from build123d import *

# Parameters (mm, degrees)
SKETCH1_R           = 13
BOSS_EXTRUDE1_DEPTH = 10
SKETCH3_R           = 17
BOSS_EXTRUDE2_DEPTH = 1
CUT_EXTRUDE2_DEPTH  = 27.438608133


with BuildPart() as part:
    # Sketch1 → Boss-Extrude1 (new body)
    with BuildSketch(Plane(origin=(0, 0, 0), x_dir=(1, 0, 0), z_dir=(0, 1, 0))):
        with Locations(Location((0, 0, 0), (0, 0, 270))):
            Circle(SKETCH1_R)
    extrude(amount=BOSS_EXTRUDE1_DEPTH)

    # Sketch2 → Cut-Revolve1 (revolve, cut)
    with BuildSketch(Plane(origin=(0, 0, 0), x_dir=(0, 0, -1), z_dir=(1, 0, 0)), mode=Mode.PRIVATE) as cut_revolve1_sk:
        Polygon((-13, 0), (-10.757403894, 10), (-13, 10), align=None)
    revolve(cut_revolve1_sk.sketch.rotate(Axis((0, 0, 0), (0, 1, 0)), 180), axis=Axis((0, 0, 0), (0, 1, 0)), mode=Mode.SUBTRACT)

    # Sketch3 → Boss-Extrude2 (add)
    with BuildSketch(Plane(origin=(0, 0, 0), x_dir=(-1, 0, 0), z_dir=(0, -1, 0))):
        with Locations(Location((0, 0, 0), (0, 0, 90))):
            Circle(SKETCH3_R)
    extrude(amount=BOSS_EXTRUDE2_DEPTH)

    # Sketch5 → Cut-Extrude2 (cut, through all)
    with BuildSketch(Plane(origin=(0, 10, 0), x_dir=(1, 0, 0), z_dir=(0, 1, 0))):
        with BuildLine():
            Line((1.322875656, 1.5), (-1.322875656, 1.5))
            ThreePointArc((-1.322875656, 1.5), (-0.822875656, -1.822875656), (2, 0))
            ThreePointArc((2, 0), (1.822875656, 0.822875656), (1.322875656, 1.5))
        make_face()
    extrude(amount=-CUT_EXTRUDE2_DEPTH, mode=Mode.SUBTRACT)


solid = part.part
Can you work these out from the model? Positions are in its coordinate system, mm. A direction names the side the tool comes from. Round coordinates to 2 decimals unless told otherwise and drop trailing zeros. Order: outer loops, then holes, each group sorted by start corner. A loop starts at its lowest first (then second) coordinate and runs counter-clockwise, first axis right, second up. Notation, with made-up numbers: M 26.25,12.25 L 34.25,12.25 A33 cw 34.25,48.25 Z; hole C 47,-20.5 d3. An arc over 180 degrees is marked long. Use a Markdown table: item, result.
1) I'm going to push flat-ended pins straight in: P1, Ø3.5, axis at x = 0, z = 0, coming from the +Y side; P2, Ø6, axis at y = 8.5, z = -9.5, coming from the +X side; P3, Ø3, axis at x = -0.5, y = 5.5, coming from the +Z side; P4, Ø1, axis at x = 9, y = 7, coming from the +Z side. Where does each tip first touch, or does it pass through?
Geometry says:
| item | result |
|---|---|
| P1 | stops at y = 10 |
| P2 | stops at x = 9.14 |
| P3 | stops at z = 12.1 |
| P4 | stops at z = 7.67 |
2) If I drill on line 1 along Y through (x, z) = (11, 9.5); line 2 along X through (y, z) = (5.5, 0.5); line 3 along Z through (x, y) = (9, 5), over which ranges is the centre line in solid material (lowest first)?
Geometry says:
| item | result |
|---|---|
| line 1 | y = -1 to 0 |
| line 2 | x = -11.76 to -1.94, 1.94 to 11.76 |
| line 3 | z = -7.75 to 7.75 |
3) Imagine slicing it at C-C (x = 13.5). List the corners of the cut face in (y, z) for me.
Geometry says:
| item | result |
|---|---|
| outline | M -1,-10.33 L 0,-10.33 L 0,10.33 L -1,10.33 Z |
4) On a 3-axis mill with a long thin cutter (end or side, diameter ignored), from which of +Z, -Z, +X, -X, +Y, -Y can I reach the whole of each face in a straight line? I mean faces 1 (the face through (-13, 0, 4)), 2 (the face through (-2.2, 10, -0.2)). Say none if no direction works.
Geometry says:
| item | result |
|---|---|
| face 1 | +Y |
| face 2 | +Z, -Z, +X, -X, +Y |
5) Imagine slicing it at A-A (x = 0). List the corners of the cut face in (y, z) for me, then the cut area to 3 significant figures.
Geometry says:
| item | result |
|---|---|
| outline | M -1,-17 L 0,-17 L 0,-13 L 10,-10.76 L 10,-1.5 L -1,-1.5 Z; M -1,2 L 10,2 L 10,10.76 L 0,13 L 0,17 L -1,17 Z |
| area | 233 mm² |
6) If we mould it in two halves opening along X, with no side actions, what happens to faces 3 (the face through (0, 5, -1.5)), 4 (the face through (-4, -1, 0)), 5 (the face through (16.855, -0.493, 2.213))? For each: +X half, -X half, draft (parallel to the pull), parting line (faces both ways), or undercut.
Geometry says:
| item | result |
|---|---|
| face 3 | undercut |
| face 4 | draft |
| face 5 | parting line |
7) Imagine slicing it at D-D (z = 14.5). List the corners of the cut face in (x, y) for me.
Geometry says:
| item | result |
|---|---|
| outline | M -8.87,-1 L 8.87,-1 L 8.87,0 L -8.87,0 Z |
8) Imagine slicing it at B-B (y = 5.5). List the corners of the cut face in (x, z) for me, then the cut area to 3 significant figures.
Geometry says:
| item | result |
|---|---|
| outline | C 0,0 d23.53; hole M -1.32,-1.5 L 1.32,-1.5 A2 ccw long Z |
| area | 423 mm² |
